```python
from build123d import *

# Parameters (mm, degrees)
F0_W     = 152.4
F0_H     = 101.6
F2_DEPTH = 9.525
F4_D     = 92.075


with BuildPart() as f2:
    # F0 (on Front) → F2 (new body, symmetric)
    with BuildSketch(Plane.XZ):
        with Locations((-43.9761151315, 50.8)):
            Rectangle(F0_W, F0_H)
        with BuildLine():
            Line((-120.1761151315, 101.6), (32.2238848685, 101.6))
            ThreePointArc((32.2238848685, 101.6), (-43.9761151315, 177.8), (-120.1761151315, 101.6))
        make_face()
    extrude(amount=F2_DEPTH, both=True)

    # F4 (through all)
    with Locations(Plane.XZ.offset(25.4)):
        with Locations((-42.4015931785, 105.1330193877)):
            Hole(F4_D / 2)


solid = f2.part
```
The listing builds one solid part. Answer for the finished solid, in the listing's coordinates (mm). Round coordinates to 2 decimals unless told otherwise and drop trailing zeros. Loops run counter-clockwise (first coordinate to the right, second up) from the corner with the lowest first, then second, coordinate; pieces in that order, holes last.
Q1. Section A-A, the plane z = 126.5 is taken. Determine the outline of the cut face in (x, y) (3 decimals), then the cut area to 3 significant figures.
Q2. Find the intervals of material crossed by line 1 (X direction, y = -3.75, z = 98.5); line 2 (X direction, y = -6.25, z = 78.5); line 3 (Z direction, x = -17, y = 2), in increasing order.
Q3. Section B-B, the plane x = -23 is taken. Determine the outline of the cut face in (y, z) (3 decimals), then the cut area to 3 significant figures.
Q4. Given pin 1 Ø10 at (x, y) = (-104.5, 3.5) entering from +Z, flat-ended and moving along its own axis, determine where the tip first touches the part or whether it passes through.
Q5. Section D-D, the plane x = 8.5 is taken. Determine the outline of the cut face in (y, z) (3 decimals), then the cut area to 3 significant figures.
Q6. Section C-C, the plane y = 7.25 is taken. Determine the outline of the cut face in (x, z) (1 decimal), then the cut area to 3 significant figures.
Q7. For a pull along Z with two mould halves and no side action, classify faces 1 (the face through (-45, 9.525, 51)), 2 (the face through (-45, 0, 0)), 3 (the face through (-36.41, 0.13, 150.78)) as released by +Z, released by -Z, zero draft, split by the parting line, or undercut.
Completed:
1. outline: (-115.993, -9.525) - (-83.18, -9.525) - (-83.18, 9.525) - (-115.993, 9.525) - close; (-1.623, -9.525) - (28.041, -9.525) - (28.041, 9.525) - (-1.623, 9.525) - close
1. area: 1,190 mm2
2. line 1: x = -120.18 to -87.96, 3.16 to 32.22
2. line 2: x = -120.18 to -79.95, -4.85 to 32.22
2. line 3: z = 0 to 66.74, 143.53 to 172.87
3. outline: (-9.525, 0) - (9.525, 0) - (9.525, 63.383) - (-9.525, 63.383) - close; (-9.525, 146.883) - (9.525, 146.883) - (9.525, 174.856) - (-9.525, 174.856) - close
3. area: 1,740 mm2
4. pin 1: stops at z = 153.79
5. outline: (-9.525, 0) - (9.525, 0) - (9.525, 156.851) - (-9.525, 156.851) - close
5. area: 2,990 mm2
6. outline: (-120.2, 0) - (32.2, 0) - (32.2, 101.6) arc R76.2 ccw to (-120.2, 101.6) - close; hole circle Ø92.1 at (-42.4, 105.1)
6. area: 17,900 mm2
7. face 1: zero draft
7. face 2: released by -Z
7. face 3: undercut
